CAD build for the part. Positions are in the model's coordinates, mm. A direction names the side the tool comes from. Round coordinates to 2 decimals unless told otherwise and drop trailing zeros. Write each loop counter-clockwise with the first axis right and the second up, starting at its lowest first coordinate (ties: lowest second). Pieces come first, ordered by that corner, then holes. Notation, with made-up numbers: (-7.75, 3) -> (14.25, 3) arc R21 ccw to (14.25, 35) -> close; hole circle Ø5 at (-4, 42). An arc over 180 degrees is marked (long way). Put each result on its own line as item: value. Start each with the question number.
1. Saw through at C-C on y = 0. List the corners of the cut face in (x, z), and give its area (3 significant figures).
2. Pull direction Y, two halves, no side cores. Call faces 1 (the cylindrical face through (4.444, -20.013, 10.133)), 2 (the flat face through (-4, -21, 20)), 3 (the flat face through (-28.5, 0, 10)), 4 (the flat face through (-34, 10, 10)): pulls with the +Y half, pulls with the -Y half, needs draft (parallel to the pull), parting line crosses it, or undercut.
3. 3-axis set-ups, long thin cutter, end or side, ignore diameter. For faces 5 (the flat face through (-34, -10, 10)), 6 (the cylindrical face through (-27.29, 10.77, 9.87)), 7 (the flat face through (-35, -3.58, 8)): which of +Z, -Z, +X, -X, +Y, -Y reach the whole face in a straight line?
4. Saw through at D-D on x = 0. List the corners of the cut face in (y, z), and give its area (3 significant figures).
5. Saw through at A-A on z = 10. List the corners of the cut face in (x, y).
6. Saw through at B-B on x = -36.5. List the corners of the cut face in (y, z).
7. Flat gauge pins, fed straight in: P1, Ø5, axis at y = -10, z = 16.5, coming from the +X side; P2, Ø3, axis at x = 17.5, z = 3.5, coming from the +Y side; P3, Ø8, axis at x = -11, z = 17, coming from the -Y side. Where does each tip first touch, or does it go through?
8. Drill centre lines: line 1 (Z direction, x = -36.5, y = 6.5); line 2 (Y direction, x = -14, z = 6.25); line 3 (Y direction, x = -40.5, z = 12.25). Where is each one in solid material? Low to high. Write a range as from..to.
from build123d import *

# Parameters (mm, degrees)
F0_R         = 2.25
F2_DEPTH     = 10
F3_W         = 16
F3_H         = 7.16
F4_DEPTH     = 20.001
F5_R         = 5
F6_T2_ANGLE  = 306.799730078
F6_T4_ANGLE  = 306.799730078
F6_T10_ANGLE = 90.7011440301
F6_T12_ANGLE = 90.7011440301
F6_T14_ANGLE = 90.7011440301
F6_T16_ANGLE = 90.7011440301


# Not quite as in the source:
# - a fillet or chamfer that OpenCascade refuses, or shapes differently, is made with other operations: its cross-section is extruded or revolved along the edge and cut away or added


with BuildPart() as f1:
    # F0 (on Front) → F1 (revolve)
    with BuildSketch(Plane.XZ):
        Polygon((-20.5, 0), (-20.5, 20), (-28.5, 20), (-28.5, 10), (-28.5, 0), align=None)
    revolve(axis=Axis((0, 0, 23.8705657878), (0, 0, -1)))

    # F0 (on Front) → F2 (join, symmetric)
    with BuildSketch(Plane.XZ):
        Polygon((-20.5, 0), (-20.5, 20), (-28.5, 20), (-28.5, 10), (-28.5, 0), align=None)
        with BuildLine():
            Line((-28.5, 10), (-28.5, 20))
            Line((-28.5, 20), (-38.256097561, 17.8048780488))
            ThreePointArc((-38.256097561, 17.8048780488), (-31.5024396196, 16.2469504755), (-28.5, 10))
        make_face()
        with BuildLine():
            Line((-38.256097561, 2.1951219512), (-28.5, 0))
            Line((-28.5, 0), (-28.5, 10))
            ThreePointArc((-28.5, 10), (-31.5024396196, 3.7530495245), (-38.256097561, 2.1951219512))
        make_face()
        with BuildLine():
            ThreePointArc((-38.256097561, 2.1951219512), (-31.5024396196, 3.7530495245), (-28.5, 10))
            ThreePointArc((-28.5, 10), (-31.5024396196, 16.2469504755), (-38.256097561, 17.8048780488))
            ThreePointArc((-38.256097561, 17.8048780488), (-44.5, 10), (-38.256097561, 2.1951219512))
        make_face()
        with Locations((-36.5, 10)):
            Circle(F0_R, mode=Mode.SUBTRACT)
    extrude(amount=F2_DEPTH, both=True)

    # F3 (on face) → F4 (cut, through all)
    with BuildSketch(Plane.XY.offset(20)):
        with Locations((-36.5, 0)):
            Rectangle(F3_W, F3_H)
    extrude(amount=-F4_DEPTH, mode=Mode.SUBTRACT)

    # F5
    f5_edges = [f1.edges().sort_by_distance(p)[0] for p in [
        (-26.688012, 10, 10),
        (-26.688012, -10, 10),
    ]]
    fillet(f5_edges, radius=F5_R)

    # F6: chamfer of 0.5 on 8 edges, made by hand

    # F6_s1 → F6_t2 (revolve, cut)
    with BuildSketch(Plane(origin=(0, 0, 0), x_dir=(0, 0, 1), z_dir=(-0.447761194, -0.8941531821, 0))):
        Polygon((0.5, 28.5), (0, 28), (0, 28.5), align=None)
    revolve(axis=Axis((0, 0, 0), (0, 0, -1)), revolution_arc=F6_T2_ANGLE, mode=Mode.SUBTRACT)

    # F6_s3 → F6_t4 (revolve, cut)
    with BuildSketch(Plane(origin=(0, 0, 0), x_dir=(0, 0, 1), z_dir=(-0.447761194, -0.8941531821, 0))):
        Polygon((20, 28), (19.5, 28.5), (20, 28.5), align=None)
    revolve(axis=Axis((0, 0, 20), (0, 0, -1)), revolution_arc=F6_T4_ANGLE, mode=Mode.SUBTRACT)

    # F6_s5 → F6_t6 (revolve, cut)
    with BuildSketch(Plane.XZ):
        Polygon((-21, 20), (-20.5, 19.5), (-20.5, 20), align=None)
    revolve(axis=Axis((0, 0, 20), (0, 0, -1)), mode=Mode.SUBTRACT)

    # F6_s7 → F6_t8 (revolve, cut)
    with BuildSketch(Plane.XZ):
        Polygon((-20.5, 0.5), (-21, 0), (-20.5, 0), align=None)
    revolve(axis=Axis((0, 0, 0), (0, 0, -1)), mode=Mode.SUBTRACT)

    # F6_s9 → F6_t10 (revolve, cut)
    with BuildSketch(Plane(origin=(-29.7661054166, 15.3642741077, 0), x_dir=(0, 0, 1), z_dir=(-0.8886069942, 0.4586693906, 0))):
        Polygon((20, -5.9099383756), (19.5, -5.4099383756), (20, -5.4099383756), align=None)
    revolve(axis=Axis((-29.9541316015, 15, 20), (0, 0, 1)), revolution_arc=F6_T10_ANGLE, mode=Mode.SUBTRACT)

    # F6_s11 → F6_t12 (revolve, cut)
    with BuildSketch(Plane(origin=(-29.7661054166, -15.3642741077, 0), x_dir=(0, 0, 1), z_dir=(-0.8886069942, -0.4586693906, 0))):
        Polygon((20, 5.9099383756), (19.5, 5.4099383756), (20, 5.4099383756), align=None)
    revolve(axis=Axis((-29.9541316015, -15, 20), (0, 0, -1)), revolution_arc=F6_T12_ANGLE, mode=Mode.SUBTRACT)

    # F6_s13 → F6_t14 (revolve, cut)
    with BuildSketch(Plane(origin=(-29.7661054166, 15.3642741077, 0), x_dir=(0, 0, 1), z_dir=(-0.8886069942, 0.4586693906, 0))):
        Polygon((0.5, -5.4099383756), (0, -5.9099383756), (0, -5.4099383756), align=None)
    revolve(axis=Axis((-29.9541316015, 15, 0), (0, 0, 1)), revolution_arc=F6_T14_ANGLE, mode=Mode.SUBTRACT)

    # F6_s15 → F6_t16 (revolve, cut)
    with BuildSketch(Plane(origin=(-29.7661054166, -15.3642741077, 0), x_dir=(0, 0, 1), z_dir=(-0.8886069942, -0.4586693906, 0))):
        Polygon((0.5, 5.4099383756), (0, 5.9099383756), (0, 5.4099383756), align=None)
    revolve(axis=Axis((-29.9541316015, -15, 0), (0, 0, -1)), revolution_arc=F6_T16_ANGLE, mode=Mode.SUBTRACT)


solid = f1.part
Return value:
1. outline: (-28.5, 0) -> (-21, 0) -> (-20.5, 0.5) -> (-20.5, 19.5) -> (-21, 20) -> (-28.5, 20) -> close; (20.5, 0.5) -> (21, 0) -> (28, 0) -> (28.5, 0.5) -> (28.5, 19.5) -> (28, 20) -> (21, 20) -> (20.5, 19.5) -> close
1. area: 319 mm^2
2. face 1: undercut
2. face 2: needs draft
2. face 3: undercut
2. face 4: pulls with the +Y half
3. face 5: +Z, -Z, -X, -Y
3. face 6: +Z, -Z, -X, +Y
3. face 7: +Z, -Z, -X
4. outline: (-28.5, 0.5) -> (-28, 0) -> (-21, 0) -> (-20.5, 0.5) -> (-20.5, 19.5) -> (-21, 20) -> (-28, 20) -> (-28.5, 19.5) -> close; (20.5, 0.5) -> (21, 0) -> (28, 0) -> (28.5, 0.5) -> (28.5, 19.5) -> (28, 20) -> (21, 20) -> (20.5, 19.5) -> close
4. area: 319 mm^2
5. outline: (-44.5, -10) -> (-38.75, -10) -> (-38.75, -3.58) -> (-44.5, -3.58) -> close; (-44.5, 3.58) -> (-38.75, 3.58) -> (-38.75, 10) -> (-44.5, 10) -> close; (-34.25, -10) -> (-29.95, -10) arc R5 cw to (-25.48, -12.76) arc R28.5 ccw (long way) to (-25.48, 12.76) arc R5 cw to (-29.95, 10) -> (-34.25, 10) -> (-34.25, 3.58) -> (-28.5, 3.58) -> (-28.5, -3.58) -> (-34.25, -3.58) -> close; hole circle Ø41 at (0, 0)
6. outline: (-10, 1.8) -> (-3.58, 1.8) -> (-3.58, 7.75) -> (-10, 7.75) -> close; (-10, 12.25) -> (-3.58, 12.25) -> (-3.58, 18.2) -> (-10, 18.2) -> close; (3.58, 1.8) -> (10, 1.8) -> (10, 7.75) -> (3.58, 7.75) -> close; (3.58, 12.25) -> (10, 12.25) -> (10, 18.2) -> (3.58, 18.2) -> close
7. P1: stops at x = 27.5
7. P2: stops at y = 23.58
7. P3: stops at y = -27.63
8. line 1: z = 1.8..7.75, 12.25..18.2
8. line 2: y = -24.82..-14.97, 14.97..24.82
8. line 3: y = -10..-3.58, 3.58..10
